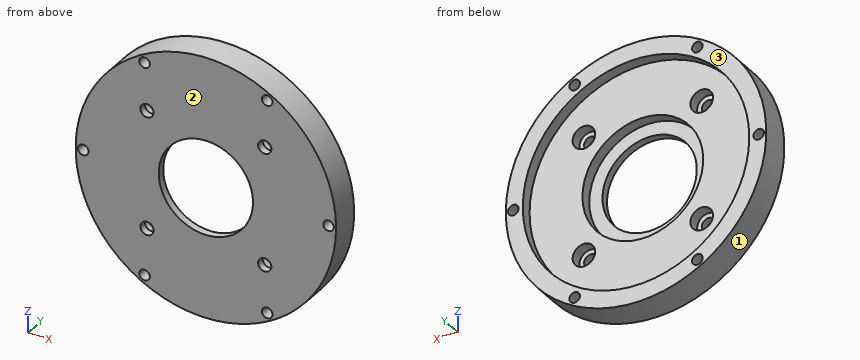
Autodesk Inventor part; units mm, degrees
ref_plane "YZ Plane" through (0, 0, 0) normal (1, 0, 0) x (0, 1, 0)
ref_plane "XZ Plane" through (0, 0, 0) normal (0, 1, 0) x (-1, 0, 0)
ref_plane "XY Plane" through (0, 0, 0) normal (0, 0, 1) x (1, 0, 0)
sketch "Sketch1" plane through (0, 0, 0) normal (0, 1, 0) x (-1, 0, 0)
  circle A0 centre (0, 0) radius 35
  dimension "d0" = 70
extrude "Extrusion1" add sketch "Sketch1" along normal blind 5
sketch "Sketch2" plane through (0, 5, 0) normal (0, 1, 0) x (1, 0, 0)
  circle A0 centre (0, 0) radius 30
  circle A1 centre (0, 0) radius 35
  dimension "d3" = 60
extrude "Extrusion2" add sketch "Sketch2" along normal blind 3
sketch "Sketch3" plane through (0, 0, 0) normal (0, -1, 0) x (1, 0, 0)
  circle A0 centre (32.5, 0) radius 1.4
  point P0 (0, 0)
  dimension "d8" = 32.5
  dimension "d9" = 2.8
extrude "Extrusion3" cut sketch "Sketch3" against normal up to surface (8 mm away)
pattern_circular "Circular Pattern1" count 6 over 360 about axis through (0, 0, 0) along (0, 1, 0) of "Extrusion3"
sketch "Sketch4" plane through (0, 0, 0) normal (0, -1, 0) x (1, 0, 0)
  circle A0 centre (0, 0) radius 12.5
  dimension "d15" = 25
extrude "Extrusion4" cut sketch "Sketch4" against normal up to surface (5 mm away)
sketch "Sketch5" plane through (0, 5, 0) normal (0, 1, 0) x (1, 0, 0)
  point P0 (0, 0)
  point P1 (-15.6, 15.6)
  point P2 (15.6, 15.6)
  point P3 (15.6, -15.6)
  point P4 (-15.6, -15.6)
  dimension "d18" = 15.6
  dimension "d19" = 15.6
  dimension "d33" = 15.6
  dimension "d34" = 15.6
hole "Hole1" at (-15.6, 5, -15.6) at (15.6, 5, -15.6) at (15.6, 5, 15.6) at (-15.6, 5, 15.6) direction (0, -1, 0) diameter 3.5 end through all
sketch "Sketch6" plane through (0, 5, 0) normal (0, 1, 0) x (1, 0, 0)
  circle A0 centre (-15.6, 15.6) radius 1.75
  circle A1 centre (-15.6, 15.6) radius 3
  point P0 (0, 0)
  dimension "d27" = 6
extrude "Extrusion5" cut sketch "Sketch6" against normal blind 3
pattern_circular "Circular Pattern2" count 4 over 360 about axis through (0, 0, 0) along (0, 1, 0) of "Extrusion5"
sketch "Sketch7" plane through (0, 5, 0) normal (0, 1, 0) x (1, 0, 0)
  circle A0 centre (0, 0) radius 16
  dimension "d35" = 32
extrude "Extrusion6" cut sketch "Sketch7" against normal blind 3
sketch "Sketch8" plane through (0, 0, 0) normal (0, -1, 0) x (1, 0, 0)
  circle A0 centre (0, 0) radius 35
  circle A1 centre (0, 0) radius 34.5
  dimension "d38" = 70
  dimension "d39" = 69
extrude "Extrusion7" cut sketch "Sketch8" against normal up to surface (8 mm away)
properties part number "Top_3DPrint"
The model under review builds one solid part; all positions refer to its coordinate system, in mm. Face numbers are marked on the shaded views. Round coordinates to 2 decimals unless told otherwise and drop trailing zeros. Order: outer loops, then holes, each group sorted by start corner. A loop starts at its lowest first (then second) coordinate and runs counter-clockwise, first axis right, second up. Notation, with made-up numbers: (30.5, 47) -> (67.5, 47) arc R18 cw to (67.5, 56) -> close; hole circle Ø2 at (2.5, -5.5). An arc over 180 degrees is marked (long way). Use a Markdown table: item, result.
Q1. We need section B-B on x = 10.5. Write out the cut boundary in (y, z), then the cut area to 3 significant figures.
Values:
| item | result |
|---|---|
| outline | (0, -32.86) -> (8, -32.86) -> (8, -28.1) -> (5, -28.1) -> (5, -12.07) -> (2, -12.07) -> (2, -6.78) -> (0, -6.78) -> close; (0, 6.78) -> (2, 6.78) -> (2, 12.07) -> (5, 12.07) -> (5, 28.1) -> (8, 28.1) -> (8, 32.86) -> (0, 32.86) -> close |
| area | 258 mm^2 |
Q2. Clearance check with flat-ended pins moving along their axes: P1, Ø5.5, axis at x = -15.6, z = 15.6, coming from the -Y side; P2, Ø3, axis at x = -13.5, y = 7, coming from the +Z side; P3, Ø7, axis at x = 15.6, z = -15.6, coming from the +Y side; P4, Ø3, axis at x = 16, z = -17, coming from the +Y side. State where each tip first meets the part, or that it passes through.
Values:
| item | result |
|---|---|
| P1 | stops at y = 0 |
| P2 | stops at z = 32.35 |
| P3 | stops at y = 5 |
| P4 | stops at y = 2 |
Q3. We need section C-C on y = 6.5. Write out the cut boundary in (x, z), then the cut area to 3 significant figures.
Values:
| item | result |
|---|---|
| outline | circle Ø69 at (0, 0); hole circle Ø2.8 at (-32.5, 0); hole circle Ø60 at (0, 0); hole circle Ø2.8 at (-16.25, -28.15); hole circle Ø2.8 at (-16.25, 28.15); hole circle Ø2.8 at (16.25, -28.15); hole circle Ø2.8 at (16.25, 28.15); hole circle Ø2.8 at (32.5, 0) |
| area | 875 mm^2 |
Q4. We need section D-D on z = -28.5. Write out the cut boundary in (x, y), then the cut area to 3 significant figures.
Values:
| item | result |
|---|---|
| outline | (-19.44, 0) -> (-17.6, 0) -> (-17.6, 8) -> (-19.44, 8) -> close; (-14.9, 0) -> (14.9, 0) -> (14.9, 8) -> (9.37, 8) -> (9.37, 5) -> (-9.37, 5) -> (-9.37, 8) -> (-14.9, 8) -> close; (17.6, 0) -> (19.44, 0) -> (19.44, 8) -> (17.6, 8) -> close |
| area | 212 mm^2 |
Q5. Mouldability with a two-part tool opening along Y and no side actions: class the marked faces 1, 2 and 3 as +Y half, -Y half, draft (parallel to the pull), parting line (faces both ways), or undercut.
Values:
| item | result |
|---|---|
| face 1 | draft |
| face 2 | -Y half |
| face 3 | +Y half |
Q6. For line 1 (X direction, y = 1.75, z = 16.5); line 2 (X direction, y = 2.25, z = 17); line 3 (Z direction, x = 0, y = 0.6), list the stretches that pass through material, from the lowest coordinate up.
Values:
| item | result |
|---|---|
| line 1 | x = -30.3 to -17.1, -14.1 to 14.1, 17.1 to 30.3 |
| line 2 | x = -30.02 to -18.25, -12.95 to 12.95, 18.25 to 30.02 |
| line 3 | z = -34.5 to -12.5, 12.5 to 34.5 |
Q7. We need section A-A on z = -3.5. Write out the cut boundary in (x, y).
Values:
| item | result |
|---|---|
| outline | (-34.32, 0) -> (-12, 0) -> (-12, 2) -> (-15.61, 2) -> (-15.61, 5) -> (-29.8, 5) -> (-29.8, 8) -> (-34.32, 8) -> close; (12, 0) -> (34.32, 0) -> (34.32, 8) -> (29.8, 8) -> (29.8, 5) -> (15.61, 5) -> (15.61, 2) -> (12, 2) -> close |
